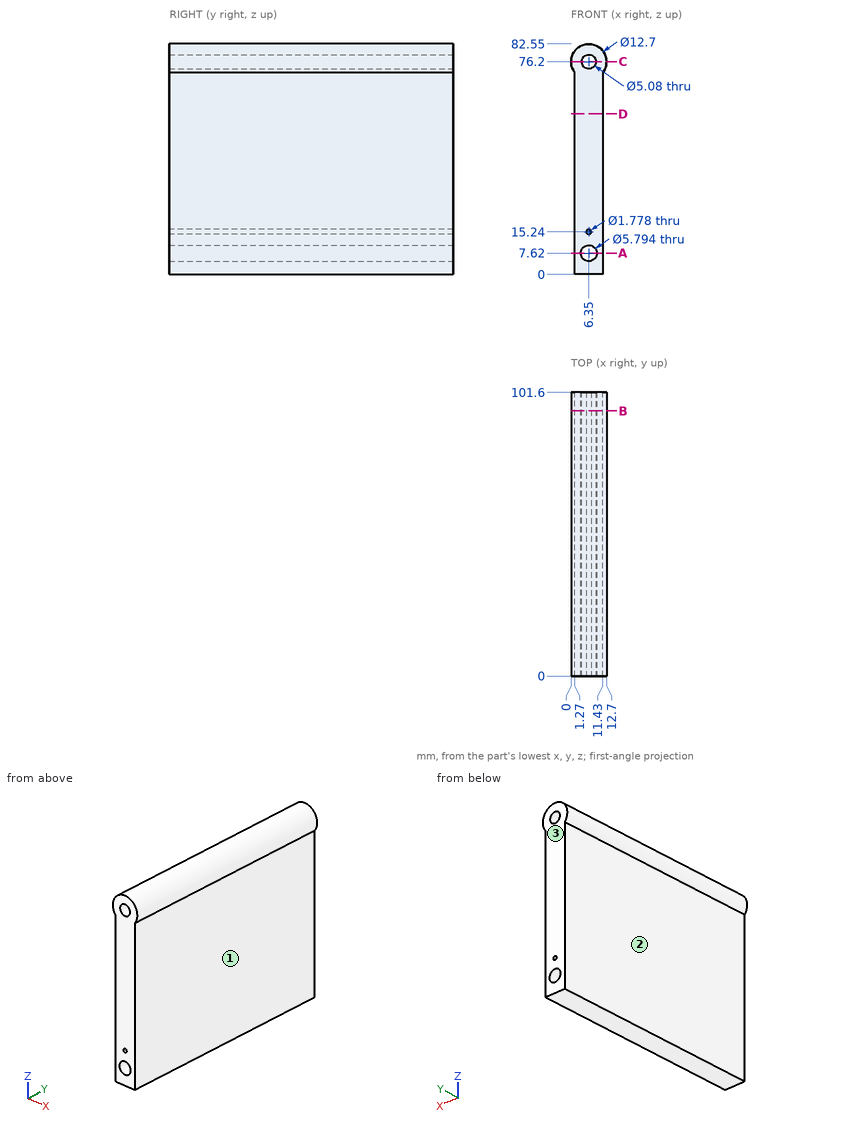
Geometry: see drawing. Coordinates: mm, zero at the bounding-box minimum. A direction names the side the tool comes from. Coordinates: 2 decimals unless noted, no trailing zeros. Loops run counter-clockwise (first coordinate to the right, second up) from the corner with the lowest first, then second, coordinate; pieces in that order, holes last.
(1) Section D-D on z = 57.5. Return the cut outline in (x, y).
(2) Section A-A on z = 7.62. Return the cut outline in (x, y).
(3) Material intervals for probe 1 along Z at (x, y) = (6.35, 65.5); probe 2 along X at (y, z) = (38, 7.5); probe 3 along Z at (x, y) = (5.25, 48.5), sorted ascending.
(4) First-contact query: pin 1 Ø21.5 at (y, z) = (55, 27.5) entering from -X; pin 2 Ø1.5 at (y, z) = (19.5, 71.5) entering from +X; pin 3 Ø5 at (x, z) = (9, 40) entering from -Y. Flat tips, straight axial feed; report the tip coordinate or a pass-through.
(5) Section C-C on z = 76.2. Return the cut outline in (x, y), then the cut area to 3 significant figures.
(6) Section B-B on y = 95. Return the cut outline in (x, z).
(7) Set-up query: the marked faces 1, 2 and 3. Return all of +Z, -Z, +X, -X, +Y, -Y with unobstructed straight access to the full face (end or side cutting, diameter ignored); none if empty.
Data:
1. outline: (1.27, 0) - (11.43, 0) - (11.43, 101.6) - (1.27, 101.6) - close
2. outline: (1.27, 0) - (3.45, 0) - (3.45, 101.6) - (1.27, 101.6) - close; (9.25, 0) - (11.43, 0) - (11.43, 101.6) - (9.25, 101.6) - close
3. probe 1: z = 0 to 4.72, 10.52 to 14.35, 16.13 to 73.66, 78.74 to 82.55
3. probe 2: x = 1.27 to 3.46, 9.24 to 11.43
3. probe 3: z = 0 to 4.94, 10.3 to 73.91, 78.49 to 82.45
4. pin 1: stops at x = 1.27
4. pin 2: stops at x = 11.43
4. pin 3: stops at y = 0
5. outline: (0, 0) - (3.81, 0) - (3.81, 101.6) - (0, 101.6) - close; (8.89, 0) - (12.7, 0) - (12.7, 101.6) - (8.89, 101.6) - close
5. area: 774 mm2
6. outline: (1.27, 0) - (11.43, 0) - (11.43, 72.39) arc R6.35 ccw (long way) to (1.27, 72.39) - close; hole circle Ø5.79 at (6.35, 7.62); hole circle Ø5.08 at (6.35, 76.2); hole circle Ø1.78 at (6.35, 15.24)
7. face 1: -Z, +X, +Y, -Y
7. face 2: -Z, -X, +Y, -Y
7. face 3: +Z, -Z, +X, -X, +Y
